Check sheet for the modelled part. Datum: model origin and axes. Units: mm. Face numbers are marked on the shaded views. Round coordinates to 2 decimals unless told otherwise and drop trailing zeros. Order: outer loops, then holes, each group sorted by start corner. A loop starts at its lowest first (then second) coordinate and runs counter-clockwise, first axis right, second up.
Q1. Cross-section at A-A on x = 95.25. Record the cut outline in (y, z).
Q2. Depth check by flat-ended pin: P1, Ø1.5, axis at y = 5.5, z = -41, coming from the -X side. Enter the tip coordinate at first touch or a pass-through.
Q3. Mould release check, pull along Z, two halves, no side actions. Record for the marked faces 1, 2 and 3: +Z half, -Z half, draft (parallel to the pull), parting line (faces both ways), or undercut.
Q4. Scan lines: probe 1 along X at (y, z) = (12.5, -95.25); probe 2 along Z at (x, y) = (95, 8); probe 3 along Z at (x, y) = (4, 11). Record each from-to range of solid material in increasing order.
Q5. Cross-section at B-B on z = -95.25. Record the cut outline in (x, y).
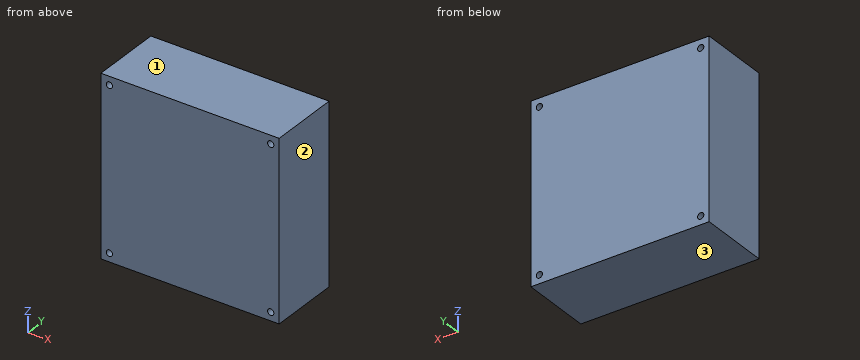
from build123d import *

# Parameters (mm, degrees)
ESBO_O1_W                = 100
ESBO_O1_H                = 100
ESBO_O1_R                = 1.75
RESSALTO_EXTRUS_O1_DEPTH = 40


with BuildPart() as part:
    # Esboço1 → Ressalto-extrusão1 (new body)
    with BuildSketch(Plane(origin=(0, 40, 0), x_dir=(1, 0, 0), z_dir=(0, 1, 0))):
        with Locations((50, 50)):
            Rectangle(ESBO_O1_W, ESBO_O1_H)
        with Locations(Location((4.75, 95.25, 0), (0, 0, 90))):
            Circle(ESBO_O1_R, mode=Mode.SUBTRACT)
        with Locations(Location((95.25, 95.25, 0), (0, 0, 90))):
            Circle(ESBO_O1_R, mode=Mode.SUBTRACT)
        with Locations(Location((95.25, 4.75, 0), (0, 0, 90))):
            Circle(ESBO_O1_R, mode=Mode.SUBTRACT)
        with Locations(Location((4.75, 4.75, 0), (0, 0, 90))):
            Circle(ESBO_O1_R, mode=Mode.SUBTRACT)
    extrude(amount=-RESSALTO_EXTRUS_O1_DEPTH)


solid = part.part
Results found:
1. outline: (0, -100) - (40, -100) - (40, -97) - (0, -97) - close; (0, -93.5) - (40, -93.5) - (40, -6.5) - (0, -6.5) - close; (0, -3) - (40, -3) - (40, 0) - (0, 0) - close
2. P1: stops at x = 0
3. face 1: +Z half
3. face 2: draft
3. face 3: -Z half
4. probe 1: x = 0 to 3, 6.5 to 93.5, 97 to 100
4. probe 2: z = -100 to -96.98, -93.52 to -6.48, -3.02 to 0
4. probe 3: z = -100 to -96.83, -93.67 to -6.33, -3.17 to 0
5. outline: (0, 0) - (3, 0) - (3, 40) - (0, 40) - close; (6.5, 0) - (93.5, 0) - (93.5, 40) - (6.5, 40) - close; (97, 0) - (100, 0) - (100, 40) - (97, 40) - close
